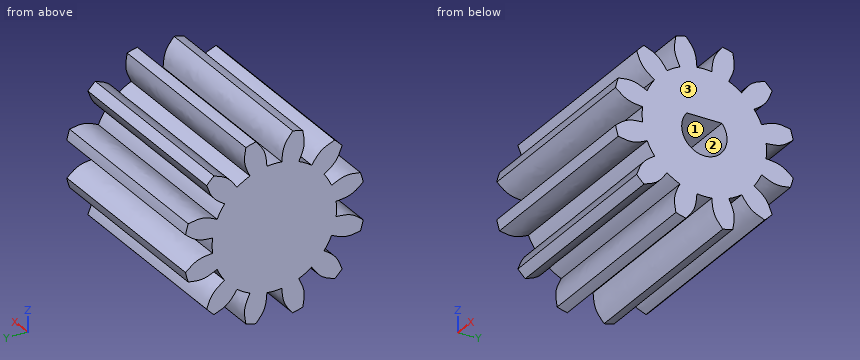
```python
from build123d import *

# Parameters (mm, degrees)
KUGGLUCKA_DEPTH    = 15
CIRPATTERN_COUNT   = 12
CUT_EXTRUDE1_START = -10
SKETCH1_R          = 4.5
CUT_EXTRUDE1_DEPTH = 10
CUT_EXTRUDE2_DEPTH = 10


with BuildPart() as part:
    # Ritning 1 → Kugghjulsämne (revolve)
    with BuildSketch(Plane.XY, mode=Mode.PRIVATE) as kugghjuls_mne_sk:
        Polygon((12.5, 1), (2.5, 1), (2.5, 3.5), (-12.5, 3.5), (-12.5, -3.5), (12.5, -3.5), align=None)
    revolve(kugghjuls_mne_sk.sketch.rotate(Axis((-12.5, -3.5, 0), (1, 0, 0)), 90), axis=Axis((-12.5, -3.5, 0), (1, 0, 0)))

    # Ritning 2 → Kugglucka (cut)
    with BuildSketch(Plane.ZY.offset(12.5)):
        with BuildLine():
            Line((1.419865071, 3.354486354), (0, 4.774351425))
            Line((0, 4.774351425), (-1.419865071, 3.354486354))
            add(Edge.make_bspline(
                [(-1.419865071, 3.354486354), (-1.173032372, 3.067088657), (-0.658113481, 2.467546927), (-0.604624671, 1.6768746), (-0.576776379, 1.265220772)],
                knots=[0, 0, 0, 0, 0.479362292, 1, 1, 1, 1], degree=3))
            ThreePointArc((-0.576776379, 1.265220772), (0, 1.3), (0.576776379, 1.265220772))
            add(Edge.make_bspline(
                [(1.419865071, 3.354486354), (1.173032372, 3.067088657), (0.658113481, 2.467546927), (0.604624671, 1.6768746), (0.576776379, 1.265220772)],
                knots=[0, 0, 0, 0, 0.479362292, 1, 1, 1, 1], degree=3))
        make_face()
    kugglucka = extrude(amount=-KUGGLUCKA_DEPTH, mode=Mode.SUBTRACT)

    # CirPattern: Kugglucka ×12 about axis
    cirpattern_axis = Axis((-12.5, -3.5, 0), (-1, 0, 0))
    for i in range(1, CIRPATTERN_COUNT):
        add(kugglucka.rotate(cirpattern_axis, i * 360 / CIRPATTERN_COUNT), mode=Mode.SUBTRACT)

    # Sketch1 → Cut-Extrude1 (cut)
    with BuildSketch(Plane(origin=(12.5, 0, 0), x_dir=(0, 0, -1), z_dir=(1, 0, 0)).offset(CUT_EXTRUDE1_START)):
        with Locations((0, -3.5)):
            Circle(SKETCH1_R)
    extrude(amount=CUT_EXTRUDE1_DEPTH, mode=Mode.SUBTRACT)

    # Sketch2 → Cut-Extrude2 (cut)
    with BuildSketch(Plane(origin=(2.5, 0, 0), x_dir=(0, 0, -1), z_dir=(1, 0, 0))):
        with BuildLine():
            Line((-1.1, -2.138934241), (-1.1, -4.861065759))
            ThreePointArc((-1.1, -4.861065759), (1.75, -3.5), (-1.1, -2.138934241))
        make_face()
    extrude(amount=-CUT_EXTRUDE2_DEPTH, mode=Mode.SUBTRACT)


solid = part.part
```
Geometry check sheet. Reference: the model listing, model coordinates, mm. Face numbers are marked on the shaded views. Give positions to 0.01 mm unless a question says otherwise; leave off trailing zeros. Loops run counter-clockwise (first coordinate to the right, second up) from the corner with the lowest first, then second, coordinate; pieces in that order, holes last. Notation, with made-up numbers: M 1,-37 L 27,-37 A27 ccw 27,-2 Z; hole C 42.25,-4 d3. An arc over 180 degrees is marked long. Write item = value, one per line.
(1) Sectioned sample at A-A, the plane z = 0. Record the cut outline in (x, y), plus the area to 3 significant figures.
Answer below:
outline = M -12.5,-8.3 L 2.5,-8.3 L 2.5,-5.25 L -7.5,-5.25 L -7.5,-1.75 L 2.5,-1.75 L 2.5,1.3 L -12.5,1.3 Z
area = 109 mm2
(2) Gauge pin test, flat ends, axial feed: pin 1 Ø5 at (x, y) = (-3, -2) entering from +Z; pin 2 Ø0.9 at (y, z) = (-4.5, -0.5) entering from +X. Record the tip position at first contact, or that the pin passes through.
Answer below:
pin_1 = 6.85
pin_2 = -7.5
(3) Release check for a two-part mould opening along Y. For the marked faces 1, 2 and 3 record: released by +Y, released by -Y, zero draft, split by the parting line, or undercut.
Answer below:
face_1 = undercut
face_2 = undercut
face_3 = zero draft
(4) Material ranges on line 1 (Y direction, x = -1.75, z = 0); line 2 (Y direction, x = 1.25, z = 4); line 3 (Z direction, x = -3.5, y = -3.5), recorded low to high. Write a range as [from, to].
Answer below:
line_1 = [-8.3, -5.25], [-1.75, 1.3]
line_2 = [-8.47, -6.49], [-6.15, -0.85], [-0.51, 1.47]
line_3 = [-4.8, -1.75], [1.1, 4.8]
(5) Sectioned sample at B-B, the plane y = -3.5. Record the cut outline in (x, z).
Answer below:
outline = M -12.5,-4.8 L 2.5,-4.8 L 2.5,-1.75 L -7.5,-1.75 L -7.5,1.1 L 2.5,1.1 L 2.5,4.8 L -12.5,4.8 Z
